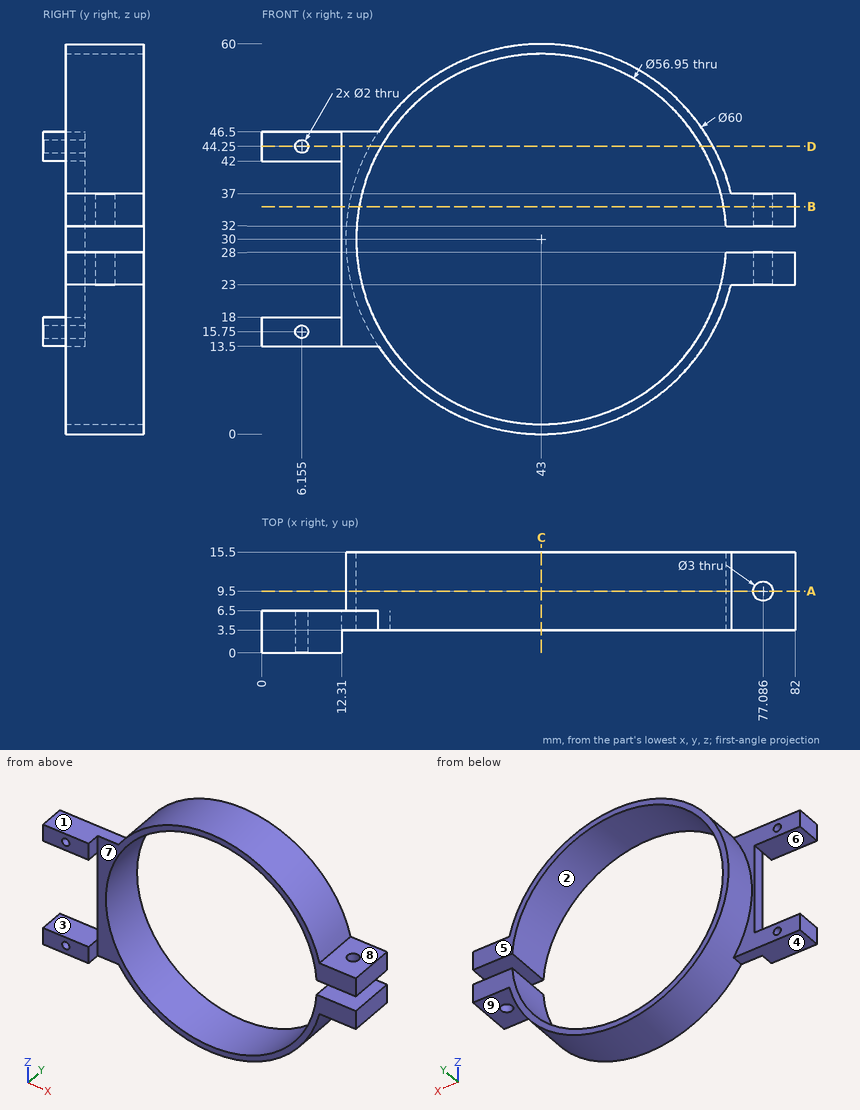
Could you check a few things on this drawing? It's one solid part, dimensions in mm from its lowest x, y, z. A direction names the side the tool comes from. Round coordinates to 2 decimals unless told otherwise and drop trailing zeros. Write each loop counter-clockwise with the first axis right and the second up, starting at its lowest first coordinate (ties: lowest second). Pieces come first, ordered by that corner, then holes. Notation, with made-up numbers: (72, -33) -> (119, -33) arc R33 ccw to (119, -4) -> close; hole circle Ø10 at (-18.5, 83.25). An arc over 180 degrees is marked (long way). Use one line per item in the form item = value. Start each with the question number.
Q1. Imagine slicing it at C-C (x = 43). Please give me the cut outline in (y, z) (3 decimals).
Q2. Imagine slicing it at A-A (y = 9.5). Please give me the cut outline in (x, z) (3 decimals).
Q3. Imagine slicing it at B-B (z = 35). Please give me the cut outline in (x, y).
Q4. If I drill on probe 1 along X at (y, z) = (9.5, 34.7); probe 2 along X at (y, z) = (5.25, 44.25) (1 decimal); probe 3 along Z at (x, y) = (42, 12.25), over which ranges is the centre line in solid material (lowest first)? Write a range as [from, to].
Q5. We'd pull the mould along Z, two halves only. Please class the marked faces 1, 2, 3 and 4: +Z half, -Z half, draft (parallel to the pull), parting line (faces both ways), or undercut.
Q6. Which directions (+Z, -Z, +X, -X, +Y, -Y) give clear straight access to the entire face, cutting with the end or side of a thin tool? Please do the marked faces 5, 6, 7, 8 and 9.
Q7. Imagine slicing it at D-D (z = 44.25). Please give me the cut outline in (x, y) (1 decimal), then the cut area to 3 significant figures.
Q8. I'm going to push flat-ended pins straight in: P1, Ø6, axis at x = 73, y = 8.5, coming from the -Z side; P2, Ø1.5, axis at x = 39.5, y = 8.5, coming from the +Z side; P3, Ø1, axis at y = 5, z = 52.5, coming from the +X side; P4, Ø5, axis at y = 8.5, z = 37.5, coming from the +X side. Where does each tip first touch, or does it pass through?
Worked out:
q1.outline = (3.5, 0) -> (15.5, 0) -> (15.5, 1.525) -> (3.5, 1.525) -> close; (3.5, 58.475) -> (15.5, 58.475) -> (15.5, 60) -> (3.5, 60) -> close
q2.outline = (71.405, 28) arc R28.475 cw (long way) to (71.405, 32) -> (75.586, 32) -> (75.586, 37) -> (72.172, 37) arc R30 ccw (long way) to (72.172, 23) -> (75.586, 23) -> (75.586, 28) -> close; (78.586, 23) -> (82, 23) -> (82, 28) -> (78.586, 28) -> close; (78.586, 32) -> (82, 32) -> (82, 37) -> (78.586, 37) -> close
q3.outline = (12.31, 3.5) -> (14.97, 3.5) -> (14.97, 15.5) -> (13.42, 15.5) -> (13.42, 6.5) -> (12.31, 6.5) -> close; (71.03, 3.5) -> (82, 3.5) -> (82, 15.5) -> (71.03, 15.5) -> close; hole circle Ø3 at (77.09, 9.5)
q4.probe_1 = [13.37, 14.92], [71.08, 75.59], [78.59, 82]
q4.probe_2 = [0, 5.2], [7.2, 18.3], [67.7, 69.4]
q4.probe_3 = [0.02, 1.54], [58.46, 59.98]
q5.face_1 = +Z half
q5.face_2 = undercut
q5.face_3 = undercut
q5.face_4 = -Z half
q6.face_5 = +Z, -Z, +X, -X, +Y
q6.face_6 = -X, +Y, -Y
q6.face_7 = +Z, -Z, +X, -Y
q6.face_8 = +Z, +X, +Y, -Y
q6.face_9 = -Z, +X, +Y, -Y
q7.outline = (0, 0) -> (5.2, 0) -> (5.2, 6.5) -> (0, 6.5) -> close; (7.2, 0) -> (12.3, 0) -> (12.3, 3.5) -> (18.3, 3.5) -> (18.3, 15.5) -> (16.6, 15.5) -> (16.6, 6.5) -> (7.2, 6.5) -> close; (67.7, 3.5) -> (69.4, 3.5) -> (69.4, 15.5) -> (67.7, 15.5) -> close
q7.area = 122 mm^2
q8.P1 = 16.92
q8.P2 = 59.87
q8.P3 = 63.4
q8.P4 = 82
